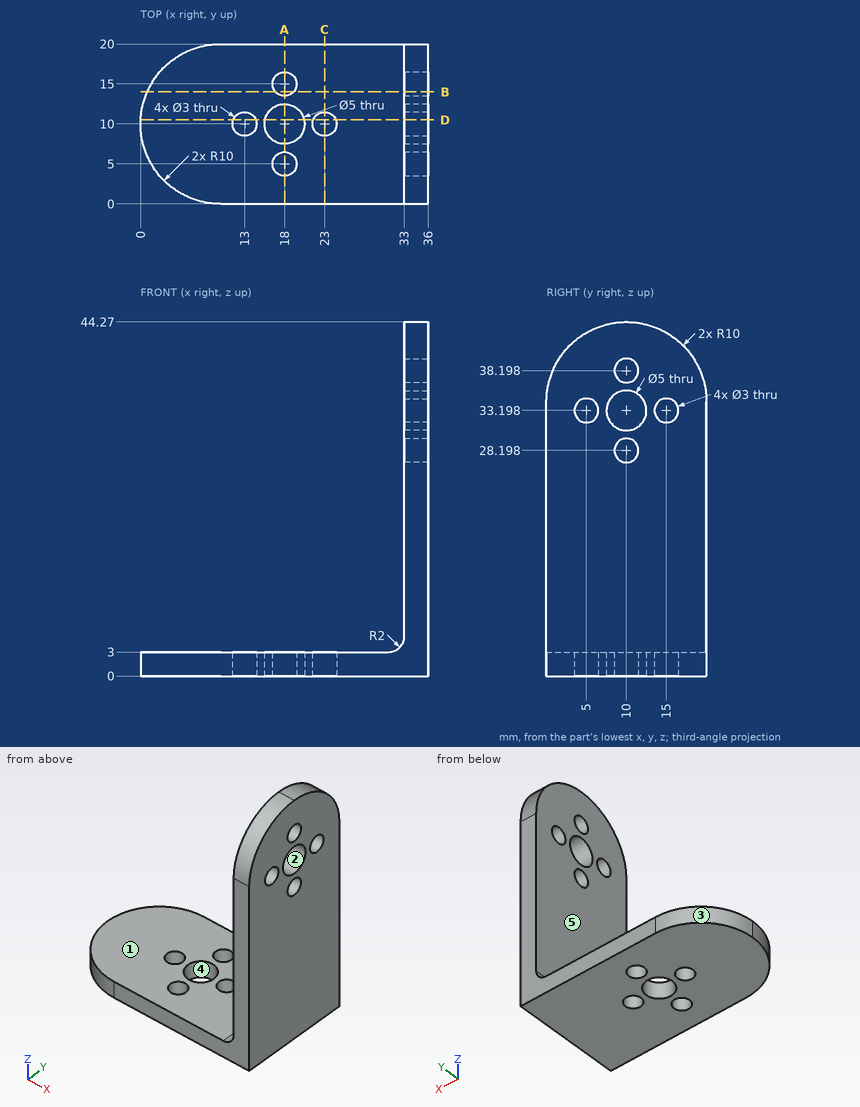
Here's the drawing with two shaded views (mm, measured from the low corner). I have some questions. A direction names the side the tool comes from. Give positions to 0.01 mm unless a question says otherwise; leave off trailing zeros. Write each loop counter-clockwise with the first axis right and the second up, starting at its lowest first coordinate (ties: lowest second). Pieces come first, ordered by that corner, then holes. Notation, with made-up numbers: (31, 33.5) -> (76, 33.5) arc R5 cw to (76, 40.5) -> close; hole circle Ø10 at (-9, -37). An arc over 180 degrees is marked (long way). Answer as a JSON object with one key per item and string values. Group by question number.
Item 1: Suppose I cut it at D-D (y = 10.5). State how many separate pieces and enclosed holes the cut face has, plus the area to 3 significant figures.
Item 2: Suppose I cut it at A-A (x = 18). Please give me the cut outline in (y, z).
Item 3: For the marked faces 1 and 2, which set-ups out of +Z, -Z, +X, -X, +Y, -Y let a thin tool reach every point of the face, with its end or its side?
Item 4: Suppose I cut it at B-B (y = 14). Please give me the cut outline in (x, z) (3 decimals), plus the area to 3 significant figures.
Item 5: We'd pull the mould along Y, two halves only. Please class the marked faces 3, 4 and 5: +Y half, -Y half, draft (parallel to the pull), parting line (faces both ways), or undercut.
Item 6: Suppose I cut it at C-C (x = 23). Please give me the cut outline in (y, z).
Item 7: I'm going to push flat-ended pins straight in: P1, Ø10, axis at y = 5.5, z = 20, coming from the -X side; P2, Ø10, axis at x = 25, y = 12, coming from the +Z side; P3, Ø1, axis at y = 10, z = 33, coming from the -X side. Where does each tip first touch, or does it pass through?
Item 8: Please list where these lines run through material, in increasing order: line 1 (Y direction, x = 18, z = 0.8); line 2 (Z direction, x = 10.5, y = 5.5); line 3 (Y direction, x = 13, z = 1). Write a range as [from, to].
Findings:
{
 "1": {"separate pieces": "7", "enclosed holes": "0", "area": "169 mm²"},
 "2": {"outline": "(0, 0) -> (3.5, 0) -> (3.5, 3) -> (0, 3) -> close; (6.5, 0) -> (7.5, 0) -> (7.5, 3) -> (6.5, 3) -> close; (12.5, 0) -> (13.5, 0) -> (13.5, 3) -> (12.5, 3) -> close; (16.5, 0) -> (20, 0) -> (20, 3) -> (16.5, 3) -> close"},
 "3": {"face 1": "+Z, -X, +Y, -Y", "face 2": "+X, -X"},
 "4": {"outline": "(0.835, 0) -> (16.882, 0) -> (16.882, 3) -> (0.835, 3) -> close; (19.118, 0) -> (36, 0) -> (36, 32.08) -> (33, 32.08) -> (33, 5) arc R2 cw to (31, 3) -> (19.118, 3) -> close; (33, 34.316) -> (36, 34.316) -> (36, 43.435) -> (33, 43.435) -> close", "area": "214 mm²"},
 "5": {"face 3": "+Y half", "face 4": "undercut", "face 5": "draft"},
 "6": {"outline": "(0, 0) -> (8.5, 0) -> (8.5, 3) -> (0, 3) -> close; (11.5, 0) -> (20, 0) -> (20, 3) -> (11.5, 3) -> close"},
 "7": {"P1": "stops at x = 33", "P2": "stops at z = 3", "P3": "passes through"},
 "8": {"line 1": "y = [0, 3.5], [6.5, 7.5], [12.5, 13.5], [16.5, 20]", "line 2": "z = [0, 3]", "line 3": "y = [0, 8.5], [11.5, 20]"}
}
